Verification items for the finished model (mm, model axes). Coordinates: 2 decimals unless noted, no trailing zeros. Order: outer loops, then holes, each group sorted by start corner. A loop starts at its lowest first (then second) coordinate and runs counter-clockwise, first axis right, second up. Notation, with made-up numbers: (-33.5, -33.5) -> (-22.5, -33.5) arc R9 ccw to (-22.5, -20.5) -> close; hole circle Ø6 at (10, 9). An arc over 180 degrees is marked (long way). Answer as CSV lines item,"result".
```python
from build123d import *

# Parameters (mm, degrees)
BOSS_EXTRUDE1_DEPTH = 3.175


with BuildPart() as part:
    # Sketch2 → Boss-Extrude1 (new body)
    with BuildSketch(Plane(origin=(0, 0, 0), x_dir=(1, 0, 0), z_dir=(0, 1, 0))):
        with BuildLine():
            Line((-1.5113, -19.05), (-1.5113, -9.6012))
            Line((-1.5113, -9.6012), (1.5113, -9.6012))
            Line((1.5113, -9.6012), (1.5113, -19.05))
            Line((1.5113, -19.05), (6.35, -19.05))
            Line((6.35, -19.05), (101.892440563, -43.858854449))
            ThreePointArc((101.892440563, -43.858854449), (105.652252874, -41.929489283), (104.164919451, -37.973926385))
            Line((104.164919451, -37.973926385), (32.442533737, -0.363160318))
            ThreePointArc((32.442533737, -0.363160318), (31.727309935, -0.092126666), (30.968022767, 0))
            Line((30.968022767, 0), (25.4762, 0))
            Line((25.4762, 0), (25.4762, 3.2512))
            Line((25.4762, 3.2512), (12.6238, 3.2512))
            Line((12.6238, 3.2512), (12.6238, 0))
            Line((12.6238, 0), (6.4262, 0))
            Line((6.4262, 0), (6.4262, 3.2512))
            Line((6.4262, 3.2512), (-6.4262, 3.2512))
            Line((-6.4262, 3.2512), (-6.4262, 0))
            Line((-6.4262, 0), (-12.6238, 0))
            Line((-12.6238, 0), (-12.6238, 3.2512))
            Line((-12.6238, 3.2512), (-25.4762, 3.2512))
            Line((-25.4762, 3.2512), (-25.4762, 0))
            Line((-25.4762, 0), (-30.95625, 0))
            ThreePointArc((-30.95625, 0), (-31.726300609, -0.094797562), (-32.450367647, -0.373529412))
            Line((-32.450367647, -0.373529412), (-103.023886624, -38.012739533))
            ThreePointArc((-103.023886624, -38.012739533), (-104.485708905, -41.973107934), (-100.721752751, -43.884671777))
            Line((-100.721752751, -43.884671777), (-6.35, -19.05))
            Line((-6.35, -19.05), (-1.5113, -19.05))
        make_face()
        with BuildLine():
            Line((-52.083424577, -18.041159774), (-30.862867647, -6.723529412))
            ThreePointArc((-30.862867647, -6.723529412), (-30.138800609, -6.444797562), (-29.36875, -6.35))
            Line((-29.36875, -6.35), (-11.126341516, -6.35))
            ThreePointArc((-11.126341516, -6.35), (-8.876399737, -7.28482434), (-7.951371556, -9.538811345))
            Line((-7.951371556, -9.538811345), (-7.955433254, -10.472519677))
            ThreePointArc((-7.955433254, -10.472519677), (-8.620060106, -12.402622549), (-10.322386989, -13.529169988))
            Line((-10.322386989, -13.529169988), (-49.781290705, -23.913092018))
            ThreePointArc((-49.781290705, -23.913092018), (-53.545246858, -22.001528175), (-52.083424577, -18.041159774))
        make_face(mode=Mode.SUBTRACT)
        with BuildLine():
            Line((7.941592001, -9.529086738), (7.942778948, -10.451228904))
            ThreePointArc((7.942778948, -10.451228904), (8.607635671, -12.39131781), (10.3198084, -13.520230548))
            Line((10.3198084, -13.520230548), (50.025691322, -23.830386583))
            ThreePointArc((50.025691322, -23.830386583), (53.785503632, -21.901021417), (52.29817021, -17.945458519))
            Line((52.29817021, -17.945458519), (30.878579271, -6.713160318))
            ThreePointArc((30.878579271, -6.713160318), (30.163355469, -6.442126666), (29.404068301, -6.35))
            Line((29.404068301, -6.35), (11.116589371, -6.35))
            ThreePointArc((11.116589371, -6.35), (8.870080926, -7.281381315), (7.941592001, -9.529086738))
        make_face(mode=Mode.SUBTRACT)
    extrude(amount=BOSS_EXTRUDE1_DEPTH)


solid = part.part
```
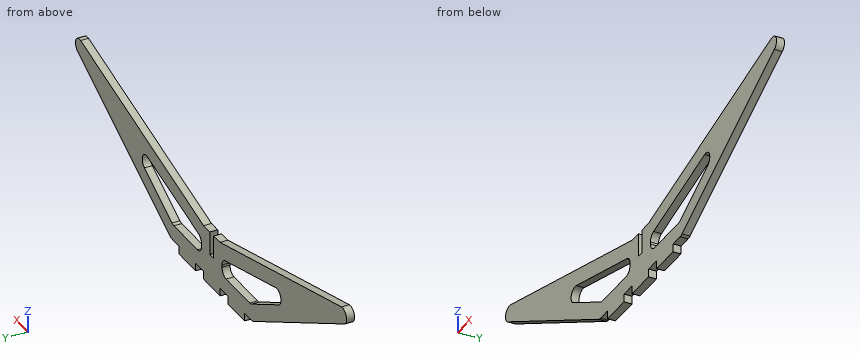
Item 1: Depth check by flat-ended pin: pin 1 Ø1.6 at (y, z) = (2, -2.5) entering from +X; pin 2 Ø1 at (x, y) = (11, 1) entering from -Z; pin 3 Ø1 at (y, z) = (1, -1.5) entering from -X. Enter the tip coordinate at first touch or a pass-through.
Answer list:
pin 1,"x = 25.48"
pin 2,"z = 0"
pin 3,"x = -25.48"
Item 2: Thickness scan on line 1 (Z direction, x = -40.5, y = 2.1); line 2 (Z direction, x = -44.5, y = 2.75); line 3 (Z direction, x = 6, y = 2.9). Record the ranges inside material, lowest first.
Answer list:
line 1,"4.67 to 11.86, 21.47 to 28.04"
line 2,"6.8 to 14, 22.52 to 29.09"
line 3,"-3.25 to 19.05"
Item 3: Section check B-B, the plane x = 21. Record the boundary of the cut face in (y, z) (3 decimals).
Answer list:
outline,"(0, -3.251) -> (3.175, -3.251) -> (3.175, 6.35) -> (0, 6.35) -> close; (0, 16.293) -> (3.175, 16.293) -> (3.175, 22.854) -> (0, 22.854) -> close"
Item 4: Section check C-C, the plane z = 16. Record the boundary of the cut face in (x, y) (3 decimals), plus the area to 3 significant figures.
Answer list:
outline,"(-61.75, 0) -> (-48.256, 0) -> (-48.256, 3.175) -> (-61.75, 3.175) -> close; (-19.712, 0) -> (-1.511, 0) -> (-1.511, 3.175) -> (-19.712, 3.175) -> close; (1.511, 0) -> (19.87, 0) -> (19.87, 3.175) -> (1.511, 3.175) -> close; (48.588, 0) -> (62.261, 0) -> (62.261, 3.175) -> (48.588, 3.175) -> close"
area,"202 mm2"
Item 5: Section check A-A, the plane z = 40. Record the boundary of the cut face in (x, y) (3 decimals).
Answer list:
outline,"(-104.599, 0) -> (-85.96, 0) -> (-85.96, 3.175) -> (-104.599, 3.175) -> close; (87.031, 0) -> (105.767, 0) -> (105.767, 3.175) -> (87.031, 3.175) -> close"
Item 6: Section check D-D, the plane y = 2.2. Count the separate pieces of the cut face and the enclosed holes in it, plus the area to 3 significant figures.
Answer list:
separate pieces,"1"
enclosed holes,"2"
area,"2,960 mm2"
